from build123d import *

# Parameters (mm, degrees)
SKETCH_1_R          = 2.5
EXTRUDE_1_DEPTH     = 52
CUT_EXTRUDE_START   = 37
CUT_EXTRUDE_1_DEPTH = 15
CHAMFER_1_SIZE      = 0.25


with BuildPart() as part:
    # 草图1 → 凸台-拉伸1 (new body)
    with BuildSketch(Plane(origin=(0, 0, 0), x_dir=(1, 0, 0), z_dir=(0, 1, 0))):
        with Locations(Location((0, 0, 0), (0, 0, 90))):
            Circle(SKETCH_1_R)
    extrude(amount=EXTRUDE_1_DEPTH)

    # 草图2 → 切除-拉伸1 (cut)
    with BuildSketch(Plane(origin=(0, 0, 0), x_dir=(1, 0, 0), z_dir=(0, 1, 0)).offset(CUT_EXTRUDE_START)):
        with BuildLine():
            Line((-1.5, 2), (1.5, 2))
            ThreePointArc((1.5, 2), (0, 2.5), (-1.5, 2))
        make_face()
    extrude(amount=CUT_EXTRUDE_1_DEPTH, mode=Mode.SUBTRACT)

    # 倒角1
    chamfer_1_edges = [part.edges().sort_by_distance(p)[0] for p in [
        (0, 0, 2.5),
    ]]
    chamfer(chamfer_1_edges, length=CHAMFER_1_SIZE)


solid = part.part
Here's how the part is built. I have some questions about the finished solid (model axes, mm). A direction names the side the tool comes from. Round coordinates to 2 decimals unless told otherwise and drop trailing zeros. Loops run counter-clockwise (first coordinate to the right, second up) from the corner with the lowest first, then second, coordinate; pieces in that order, holes last. Notation, with made-up numbers: (84.5, 66) - (113.5, 66) arc R26 ccw to (113.5, 101) - close; hole circle Ø2 at (25, 66). An arc over 180 degrees is marked (long way). One line per question, with ' | ' between items. Start each with the question number.
Q1. I want a section at C-C (y = 46). Write out the boundary of the cut face in (x, z).
Q2. I want a section at A-A (x = 0). Write out the boundary of the cut face in (y, z).
Q3. Will these pins go through, and if not, where does the flat tip stop? pin 1 (1 mm diameter, centred on x = -1, y = 14.5, fed in from -Z); pin 2 (1 mm diameter, centred on y = 45, z = -1, fed in from +X); pin 3 (1.5 mm diameter, centred on x = 0, y = 41.5, fed in from -Z).
Q4. For faces 1 (the flat face through (0, 44, -2)), 2 (the cylindrical face through (-0.1, 25.8, 2.5)), which set-ups out of +Z, -Z, +X, -X, +Y, -Y let a thin tool reach every point of the face, with its end or its side?
Q5. Please list where these lines run through material, in increasing order: line 1 (Z direction, x = -0.15, y = 27.5); line 2 (Z direction, x = -0.2, y = 38); line 3 (X direction, y = 32.5, z = -1.9). Write a range as [from, to].
Q6. I want a section at B-B (y = 32). Write out the boundary of the cut face in (x, z), then the cut area to 3 significant figures.
Response values:
1) outline: (-1.5, -2) - (1.5, -2) arc R2.5 ccw (long way) to start
2) outline: (0, -2.25) - (0.25, -2.5) - (37, -2.5) - (37, -2) - (52, -2) - (52, 2.5) - (0.25, 2.5) - (0, 2.25) - close
3) pin 1: stops at z = -2.45 | pin 2: stops at x = 2.45 | pin 3: stops at z = -2
4) face 1: -Z, +X, -X, +Y | face 2: +Y, -Y
5) line 1: z = [-2.5, 2.5] | line 2: z = [-2, 2.49] | line 3: x = [-1.62, 1.62]
6) outline: circle Ø5 at (0, 0) | area: 19.6 mm²
